Read the model definition and answer for the solid it produces. Units are mm, in the model's axes. A direction names the side the tool comes from. Coordinates: 2 decimals unless noted, no trailing zeros. Loops run counter-clockwise (first coordinate to the right, second up) from the corner with the lowest first, then second, coordinate; pieces in that order, holes last. Notation, with made-up numbers: (12.25, -5) - (33.25, -5) arc R33 ccw to (33.25, 24) - close; hole circle Ø7 at (80, 34). An arc over 180 degrees is marked (long way). Use one line per item in the form item = value.
from build123d import *

# Parameters (mm, degrees)
SKETCH1_R           = 2.0701
BOSS_EXTRUDE1_DEPTH = 2.286


with BuildPart() as part:
    # Sketch1 → Boss-Extrude1 (new body)
    with BuildSketch(Plane(origin=(0, 0, 0), x_dir=(-1, 0, 0), z_dir=(0, 0, -1))):
        with BuildLine():
            Line((-12.7, -29.591), (-10.541, -31.75))
            Line((-10.541, -31.75), (10.541, -31.75))
            Line((10.541, -31.75), (12.7, -29.591))
            Line((12.7, -29.591), (12.7, -3.175))
            ThreePointArc((12.7, -3.175), (13.62993597, -0.92993597), (15.875, 0))
            Line((15.875, 0), (42.291, 0))
            Line((42.291, 0), (44.45, 2.159))
            Line((44.45, 2.159), (44.45, 23.241))
            Line((44.45, 23.241), (42.291, 25.4))
            Line((42.291, 25.4), (-42.291, 25.4))
            Line((-42.291, 25.4), (-44.45, 23.241))
            Line((-44.45, 23.241), (-44.45, 2.159))
            Line((-44.45, 2.159), (-42.291, 0))
            Line((-42.291, 0), (-15.875, 0))
            ThreePointArc((-15.875, 0), (-13.62993597, -0.92993597), (-12.7, -3.175))
            Line((-12.7, -3.175), (-12.7, -29.591))
        make_face()
        with Locations((0, -12.7)):
            Circle(SKETCH1_R, mode=Mode.SUBTRACT)
        with Locations((-38.1, 12.7)):
            Circle(SKETCH1_R, mode=Mode.SUBTRACT)
        with Locations((-12.7, 12.7)):
            Circle(SKETCH1_R, mode=Mode.SUBTRACT)
        with Locations((12.7, 12.7)):
            Circle(SKETCH1_R, mode=Mode.SUBTRACT)
        with Locations((25.4, 12.7)):
            Circle(SKETCH1_R, mode=Mode.SUBTRACT)
        with Locations((38.1, 12.7)):
            Circle(SKETCH1_R, mode=Mode.SUBTRACT)
        with Locations((0, -25.4)):
            Circle(SKETCH1_R, mode=Mode.SUBTRACT)
        with Locations((0, 12.7)):
            Circle(SKETCH1_R, mode=Mode.SUBTRACT)
        with Locations((-25.4, 12.7)):
            Circle(SKETCH1_R, mode=Mode.SUBTRACT)
        Circle(SKETCH1_R, mode=Mode.SUBTRACT)
    extrude(amount=-BOSS_EXTRUDE1_DEPTH)


solid = part.part
Item 1: The part is cut by section A-A on y = 12.7. Count the separate pieces of the cut face and the enclosed holes in it, plus the area to 3 significant figures.
Results below:
separate_pieces = 8
enclosed_holes = 0
area = 137 mm²
Item 2: For a pull along Y with two mould halves and no side action, classify faces 1 (the cylindrical face through (13.65, -0.91, 1.13)), 2 (the flat face through (-12.7, -17, 1)), 3 (the flat face through (43.355, 24.336, 1.127)), 4 (the cylindrical face through (-26.513, 14.446, 1.127)) as +Y half, -Y half, draft (parallel to the pull), parting line (faces both ways), or undercut.
Results below:
face_1 = -Y half
face_2 = draft
face_3 = +Y half
face_4 = undercut
Item 3: Which of the six approach directions +Z, -Z, +X, -X, +Y, -Y give full straight-line access (tool end or side, diameter ignored) to faces 5 (the cylindrical face through (0.269, -23.348, 1.127)), 6 (the flat face through (-29, 0, 1))?
Results below:
face_5 = +Z, -Z
face_6 = +Z, -Z, -X, -Y
Item 4: The part is cut by section B-B on x = 0. Give the vertices of the cut face in (y, z).
Results below:
outline = (-31.75, 0) - (-27.47, 0) - (-27.47, 2.29) - (-31.75, 2.29) - close; (-23.33, 0) - (-14.77, 0) - (-14.77, 2.29) - (-23.33, 2.29) - close; (-10.63, 0) - (-2.07, 0) - (-2.07, 2.29) - (-10.63, 2.29) - close; (2.07, 0) - (10.63, 0) - (10.63, 2.29) - (2.07, 2.29) - close; (14.77, 0) - (25.4, 0) - (25.4, 2.29) - (14.77, 2.29) - close
Item 5: This flat-tipped pin is pushed along its axis until it touches: P1, Ø1.1, axis at y = -17, z = 1, coming from the +X side. Where does it stop, or does it pass through?
Results below:
P1 = 12.7
Item 6: Find the intervals of material crossed by L1, parallel to Y at x = 25.5, z = 1.7; L2, parallel to Y at x = 0, z = 1.65; L3, parallel to Y at x = -33, z = 1.4, in increasing order.
Results below:
L1 = 0 to 10.63, 14.77 to 25.4
L2 = -31.75 to -27.47, -23.33 to -14.77, -10.63 to -2.07, 2.07 to 10.63, 14.77 to 25.4
L3 = 0 to 25.4
Item 7: The part is cut by section C-C on x = 38.1. Give the vertices of the cut face in (y, z).
Results below:
outline = (0, 0) - (10.63, 0) - (10.63, 2.29) - (0, 2.29) - close; (14.77, 0) - (25.4, 0) - (25.4, 2.29) - (14.77, 2.29) - close
